Could you check a few things on this model? Use its own coordinates, in mm. A direction names the side the tool comes from. Round coordinates to 2 decimals unless told otherwise and drop trailing zeros. Write each loop counter-clockwise with the first axis right and the second up, starting at its lowest first coordinate (ties: lowest second). Pieces come first, ordered by that corner, then holes. Notation, with made-up numbers: M 39,3 L 57,3 A27 cw 57,41 Z; hole C 67,24.25 d10. An arc over 180 degrees is marked long. One line per item, written item: value. Start each with the question number.
(1) Which directions (+Z, -Z, +X, -X, +Y, -Y) give clear straight access to the entire face, cutting with the end or side of a thin tool? Please do faces 1 (the face through (0, -43.3, 13)), 2 (the face through (30, -1, 12)).
(2) I want a section at B-B on y = 10. Please give me the cut outline in (x, z).
(3) If I drill on L1, parallel to Y at x = 22, z = 13.25; L2, parallel to X at y = 15, z = 14.85; L3, parallel to Y at x = 16, z = 11.85, over which ranges is the centre line in solid material (lowest first)?
(4) I want a section at A-A on x = 16.5. Please give me the cut outline in (y, z), and give its area (3 significant figures).
(5) I want a section at C-C on z = 12.1. Please give me the cut outline in (x, y).
(6) Thinking about a two-plate mould opening in X: for faces 3 (the face through (-23, -32.9, 13)), 4 (the face through (29, 46, 12)), 5 (the face through (0, 43.3, 13)), 6 (the face through (-27, 7, 10)), which applies, released by +X, released by -X, zero draft, split by the parting line, or undercut?
```python
from build123d import *

# Parameters (mm, degrees)
F0_R     = 1.5
F1_DEPTH = 15
F2_W     = 50.6
F2_H     = 86.6
F2_R     = 1.5
F3_DEPTH = 22
F4_R     = 1.1
F5_DEPTH = 5
F6_W     = 105.847951
F6_H     = 180.898867
F7_DEPTH = 10


with BuildPart() as f1:
    # F0 (on Top) → F1 (new body)
    with BuildSketch(Plane.XY):
        with BuildLine():
            Line((-25, -48), (25, -48))
            ThreePointArc((25, -48), (28.535534, -46.535534), (30, -43))
            Line((30, -43), (30, 43))
            ThreePointArc((30, 43), (28.535534, 46.535534), (25, 48))
            Line((25, 48), (-27, 48))
            Line((-27, 48), (-30, 48))
            Line((-30, 48), (-30, 43))
            Line((-30, 43), (-30, -43))
            ThreePointArc((-30, -43), (-28.535534, -46.535534), (-25, -48))
        make_face()
        with Locations((-22, -36.08)):
            Circle(F0_R, mode=Mode.SUBTRACT)
        with Locations((22, -36.08)):
            Circle(F0_R, mode=Mode.SUBTRACT)
        with Locations((-22, 40)):
            Circle(F0_R, mode=Mode.SUBTRACT)
        with Locations((22, 40)):
            Circle(F0_R, mode=Mode.SUBTRACT)
    extrude(amount=F1_DEPTH)

    # F2 (on face) → F3 (cut)
    with BuildSketch(Plane.XY.offset(15)):
        Rectangle(F2_W, F2_H)
        with Locations((-22, -36.08)):
            Circle(F2_R, mode=Mode.SUBTRACT)
        with Locations((22, -36.08)):
            Circle(F2_R, mode=Mode.SUBTRACT)
        with Locations((-22, 40)):
            Circle(F2_R, mode=Mode.SUBTRACT)
        with Locations((22, 40)):
            Circle(F2_R, mode=Mode.SUBTRACT)
    extrude(amount=-F3_DEPTH, mode=Mode.SUBTRACT)

    # F4 (on face) → F5 (join)
    with BuildSketch(Plane.XY.offset(15)):
        with BuildLine():
            Line((-18.3, 43.3), (-25.3, 43.3))
            Line((-25.3, 43.3), (-25.3, 36.9))
            Line((-25.3, 36.9), (-21.3, 36.9))
            ThreePointArc((-21.3, 36.9), (-19.17868, 37.77868), (-18.3, 39.9))
            Line((-18.3, 39.9), (-18.3, 43.3))
        make_face()
        with Locations((-22, 40)):
            Circle(F4_R, mode=Mode.SUBTRACT)
        with BuildLine():
            Line((25.3, 36.9), (25.3, 43.3))
            Line((25.3, 43.3), (18.3, 43.3))
            Line((18.3, 43.3), (18.3, 39.9))
            ThreePointArc((18.3, 39.9), (19.17868, 37.77868), (21.3, 36.9))
            Line((21.3, 36.9), (25.3, 36.9))
        make_face()
        with Locations((22, 40)):
            Circle(F4_R, mode=Mode.SUBTRACT)
        with BuildLine():
            Line((18.3, -43.3), (25.3, -43.3))
            Line((25.3, -43.3), (25.3, -32.9))
            Line((25.3, -32.9), (21.3, -32.9))
            ThreePointArc((21.3, -32.9), (19.17868, -33.77868), (18.3, -35.9))
            Line((18.3, -35.9), (18.3, -43.3))
        make_face()
        with Locations((22, -36.08)):
            Circle(F4_R, mode=Mode.SUBTRACT)
        with BuildLine():
            Line((-25.3, -32.9), (-25.3, -43.3))
            Line((-25.3, -43.3), (-18.3, -43.3))
            Line((-18.3, -43.3), (-18.3, -35.9))
            ThreePointArc((-18.3, -35.9), (-19.17868, -33.77868), (-21.3, -32.9))
            Line((-21.3, -32.9), (-25.3, -32.9))
        make_face()
        with Locations((-22, -36.08)):
            Circle(F4_R, mode=Mode.SUBTRACT)
    extrude(amount=-F5_DEPTH)

    # F6 (on face) → F7 (cut)
    with BuildSketch(Plane(origin=(0, 0, 0), x_dir=(1, 0, 0), z_dir=(0, 0, -1))):
        with Locations((-5.788153, -4.893799)):
            Rectangle(F6_W, F6_H)
    extrude(amount=-F7_DEPTH, mode=Mode.SUBTRACT)


solid = f1.part
```
Found:
1. face 1: +Z, -Z
1. face 2: +Z, -Z, +X, +Y, -Y
2. outline: M -30,10 L -25.3,10 L -25.3,15 L -30,15 Z; M 25.3,10 L 30,10 L 30,15 L 25.3,15 Z
3. L1: y = -48 to -37.18, -34.98 to -32.9, 36.9 to 38.9, 41.1 to 48
3. L2: x = -30 to -25.3, 25.3 to 30
3. L3: y = -48 to -43.3, 43.3 to 48
4. outline: M -48,10 L -43.3,10 L -43.3,15 L -48,15 Z; M 43.3,10 L 48,10 L 48,15 L 43.3,15 Z
4. area: 47.0 mm²
5. outline: M -30,-43 A5 ccw -25,-48 L 25,-48 A5 ccw 30,-43 L 30,43 A5 ccw 25,48 L -30,48 Z; hole M -25.3,-32.9 L -21.3,-32.9 A3 cw -18.3,-35.9 L -18.3,-43.3 L 18.3,-43.3 L 18.3,-35.9 A3 cw 21.3,-32.9 L 25.3,-32.9 L 25.3,36.9 L 21.3,36.9 A3 cw 18.3,39.9 L 18.3,43.3 L -18.3,43.3 L -18.3,39.9 A3 cw -21.3,36.9 L -25.3,36.9 Z; hole C -22,-36.08 d2.2; hole C -22,40 d2.2; hole C 22,-36.08 d2.2; hole C 22,40 d2.2
6. face 3: undercut
6. face 4: released by +X
6. face 5: undercut
6. face 6: zero draft
